```python
from build123d import *

# Parameters (mm, degrees)
EXTRUDE_1_DEPTH = 60
EXTRUDE_2_DEPTH = 5
SKETCH_3_W      = 34
SKETCH_3_H      = 3.5
EXTRUDE_3_DEPTH = 2
EXTRUDE_4_DEPTH = 3.5
FILLET_1_R      = 2
FILLET_2_R      = 2
FILLET_3_R      = 2
FILLET_4_R      = 2


with BuildPart() as part:
    # 草图1 → 凸台-拉伸1 (new body)
    with BuildSketch(Plane.XY):
        Polygon((-6.5, -7.5), (-2.5, -7.5), (-2.5, 4), (2.5, 4), (2.5, -7.5), (6.5, -7.5), (6.5, 7.5), (-6.5, 7.5), align=None)
    extrude(amount=EXTRUDE_1_DEPTH)

    # 草图2 → 凸台-拉伸2 (add)
    with BuildSketch(Plane.ZY.offset(6.5)):
        Polygon((19, 7.5), (41, 7.5), (41, 23.906923686), (30, 33.5), (19, 23.906923686), align=None)
    extrude(amount=-EXTRUDE_2_DEPTH)

    # 草图3 → 凸台-拉伸3 (add)
    with BuildSketch(Plane(origin=(6.5, 0, 0), x_dir=(0, 0, -1), z_dir=(1, 0, 0))):
        with Locations((-30, 5.75)):
            Rectangle(SKETCH_3_W, SKETCH_3_H)
    extrude(amount=EXTRUDE_3_DEPTH)

    # 草图4 → 凸台-拉伸4 (add)
    with BuildSketch(Plane.XY.offset(47)):
        Polygon((8.5, 4), (8.5, 12), (4.795643232, 4), align=None)
    extrude_4 = extrude(amount=-EXTRUDE_4_DEPTH)

    # 镜向1: 凸台-拉伸4 across plane
    add(extrude_4.mirror(Plane.XY.offset(30)))

    # 圆角1
    fillet_1_edges = [part.edges().sort_by_distance(p)[0] for p in [
        (-4, 7.5, 41),
    ]]
    fillet(fillet_1_edges, radius=FILLET_1_R)

    # 圆角2
    fillet_2_edges = [part.edges().sort_by_distance(p)[0] for p in [
        (-4, 7.5, 19),
    ]]
    fillet(fillet_2_edges, radius=FILLET_2_R)

    # 圆角3
    fillet_3_edges = [part.edges().sort_by_distance(p)[0] for p in [
        (-4, 23.906923686, 19),
    ]]
    fillet(fillet_3_edges, radius=FILLET_3_R)

    # 圆角4
    fillet_4_edges = [part.edges().sort_by_distance(p)[0] for p in [
        (-4, 23.906923686, 41),
    ]]
    fillet(fillet_4_edges, radius=FILLET_4_R)


solid = part.part
```
Work out the finished part from the listing and answer in its coordinate system (mm). A direction names the side the tool comes from. Give positions to 0.01 mm unless a question says otherwise; leave off trailing zeros. Loops run counter-clockwise (first coordinate to the right, second up) from the corner with the lowest first, then second, coordinate; pieces in that order, holes last. Notation, with made-up numbers: (58.25, -28) -> (95.25, -28) arc R23 ccw to (95.25, -7) -> close; hole circle Ø7 at (19, 24). An arc over 180 degrees is marked (long way). One line per question, with ' | ' between items. Start each with the question number.
1) Section D-D, the plane y = 21.5 is taken. Determine the outline of the cut face in (x, z), then the cut area to 3 significant figures.
2) Each of these flat-tipped pins is pushed along its axis until it touches: pin 1 (3.5 mm diameter, centred on y = -1, z = 19.5, fed in from +X); pin 2 (0.6 mm diameter, centred on x = 7.5, y = 9.5, fed in from +Z); pin 3 (1.5 mm diameter, centred on x = -5, y = 18.5, fed in from -Z); pin 4 (4 mm diameter, centred on x = -1, z = 19.5, fed in from -Y). Where does it stop, or does it pass through?
3) Section A-A, the plane y = -1 is taken. Determine the outline of the cut face in (x, z), then the cut area to 3 significant figures.
4) Straight lines are drawn through the part: L1, parallel to X at y = 1, z = 30.5; L2, parallel to Y at x = 7, z = 41; L3, parallel to X at y = 5, z = 47.5. For each, find the intervals that lie inside material, in ascending order.
5) Section B-B, the plane z = 4 is taken. Determine the outline of the cut face in (x, y).
6) For faces 1 (the face through (1, 7.5, 30)), 2 (the face through (-4, 16, 19)), 3 (the face through (4, -7.5, 30)), 4 (the face through (7, 4, 30)), 5 (the face through (7.47, 9.78, 45.27)), determine the directions among +Z, -Z, +X, -X, +Y, -Y from which every point of the face is accessible in a straight line to the end or side of a thin tool.
7) Determine the mould class of faces 6 (the face through (-6.5, 9, 30)), 7 (the face through (2.5, -2, 30)), 8 (the face through (8.5, 6, 30)) for opening direction X: +X half, -X half, draft (parallel to the pull), parting line (faces both ways), or undercut.
8) Section C-C, the plane x = -5.25 is taken. Determine the outline of the cut face in (y, z), then the cut area to 3 significant figures.
Resolved:
1) outline: (-6.5, 19) -> (-1.5, 19) -> (-1.5, 41) -> (-6.5, 41) -> close | area: 110 mm2
2) pin 1: x = 6.5 | pin 2: z = 47 | pin 3: z = 19 | pin 4: y = -7.5
3) outline: (-6.5, 0) -> (-2.5, 0) -> (-2.5, 60) -> (-6.5, 60) -> close; (2.5, 0) -> (6.5, 0) -> (6.5, 60) -> (2.5, 60) -> close | area: 480 mm2
4) L1: -6.5 to -2.5, 2.5 to 6.5 | L2: 4 to 7.5 | L3: -6.5 to 6.5
5) outline: (-6.5, -7.5) -> (-2.5, -7.5) -> (-2.5, 4) -> (2.5, 4) -> (2.5, -7.5) -> (6.5, -7.5) -> (6.5, 7.5) -> (-6.5, 7.5) -> close
6) face 1: +Y | face 2: -Z, +X, -X, +Y | face 3: +Z, -Z, +X, -X, -Y | face 4: +Z, -Z, +X, -Y | face 5: +Z, -Z, -X, +Y
7) face 6: -X half | face 7: undercut | face 8: +X half
8) outline: (-7.5, 0) -> (7.5, 0) -> (7.5, 17) arc R2 cw to (9.5, 19) -> (23, 19) arc R2 ccw to (24.5, 19.69) -> (33.5, 30) -> (24.5, 40.31) arc R2 ccw to (23, 41) -> (9.5, 41) arc R2 cw to (7.5, 43) -> (7.5, 60) -> (-7.5, 60) -> close | area: 1,370 mm2
